from build123d import *

# Parameters (mm, degrees)
F0_W     = 103.5
F0_H     = 78.5
F0_R     = 10
F1_DEPTH = 18
F2_DEPTH = 7


with BuildPart() as f1:
    # F0 (on Top) → F1 (new body)
    with BuildSketch(Plane.XY):
        Rectangle(F0_W, F0_H)
        with Locations((-36, -24)):
            Circle(F0_R, mode=Mode.SUBTRACT)
        with Locations((-12, -24)):
            Circle(F0_R, mode=Mode.SUBTRACT)
        with Locations((12, -24)):
            Circle(F0_R, mode=Mode.SUBTRACT)
        with Locations((36, -24)):
            Circle(F0_R, mode=Mode.SUBTRACT)
        with Locations((-36, 0)):
            Circle(F0_R, mode=Mode.SUBTRACT)
        with Locations((-12, 0)):
            Circle(F0_R, mode=Mode.SUBTRACT)
        with Locations((-36, 24)):
            Circle(F0_R, mode=Mode.SUBTRACT)
        with Locations((-12, 24)):
            Circle(F0_R, mode=Mode.SUBTRACT)
        with Locations((12, 0)):
            Circle(F0_R, mode=Mode.SUBTRACT)
        with Locations((36, 0)):
            Circle(F0_R, mode=Mode.SUBTRACT)
        with Locations((12, 24)):
            Circle(F0_R, mode=Mode.SUBTRACT)
        with Locations((36, 24)):
            Circle(F0_R, mode=Mode.SUBTRACT)
    extrude(amount=F1_DEPTH)

    # F0 (on Top) → F2 (join)
    with BuildSketch(Plane.XY):
        Rectangle(F0_W, F0_H)
        with Locations((-36, -24)):
            Circle(F0_R, mode=Mode.SUBTRACT)
        with Locations((-12, -24)):
            Circle(F0_R, mode=Mode.SUBTRACT)
        with Locations((12, -24)):
            Circle(F0_R, mode=Mode.SUBTRACT)
        with Locations((36, -24)):
            Circle(F0_R, mode=Mode.SUBTRACT)
        with Locations((-36, 0)):
            Circle(F0_R, mode=Mode.SUBTRACT)
        with Locations((-12, 0)):
            Circle(F0_R, mode=Mode.SUBTRACT)
        with Locations((-36, 24)):
            Circle(F0_R, mode=Mode.SUBTRACT)
        with Locations((-12, 24)):
            Circle(F0_R, mode=Mode.SUBTRACT)
        with Locations((12, 0)):
            Circle(F0_R, mode=Mode.SUBTRACT)
        with Locations((36, 0)):
            Circle(F0_R, mode=Mode.SUBTRACT)
        with Locations((12, 24)):
            Circle(F0_R, mode=Mode.SUBTRACT)
        with Locations((36, 24)):
            Circle(F0_R, mode=Mode.SUBTRACT)
        with Locations((-36, -24)):
            Circle(F0_R)
        with Locations((-12, -24)):
            Circle(F0_R)
        with Locations((12, -24)):
            Circle(F0_R)
        with Locations((36, -24)):
            Circle(F0_R)
        with Locations((12, 0)):
            Circle(F0_R)
        with Locations((-12, 0)):
            Circle(F0_R)
        with Locations((-36, 0)):
            Circle(F0_R)
        with Locations((-36, 24)):
            Circle(F0_R)
        with Locations((-12, 24)):
            Circle(F0_R)
        with Locations((12, 24)):
            Circle(F0_R)
        with Locations((36, 24)):
            Circle(F0_R)
        with Locations((36, 0)):
            Circle(F0_R)
    extrude(amount=-F2_DEPTH)


solid = f1.part
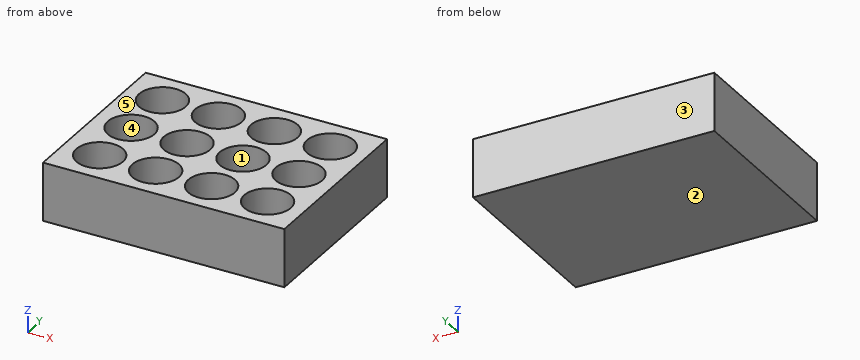
For this review, take the finished solid that the model builds, in its own axes (mm). Face numbers are marked on the shaded views. A direction names the side the tool comes from. Round coordinates to 2 decimals unless told otherwise and drop trailing zeros. Loops run counter-clockwise (first coordinate to the right, second up) from the corner with the lowest first, then second, coordinate; pieces in that order, holes last. Notation, with made-up numbers: (67, 31.5) - (124, 31.5) arc R28 ccw to (124, 68.5) - close; hole circle Ø9 at (-7, -16.75). An arc over 180 degrees is marked (long way). One line per item, written item: value. Start each with the question number.
Item 1: For L1, parallel to Y at x = -12, z = 5.75; L2, parallel to Y at x = -41.5, z = 2.5; L3, parallel to X at y = -5, z = 8, list the stretches that pass through material, from the lowest coordinate up.
Item 2: Take a section at A-A (z = 13). State how many separate pieces and enclosed holes the cut face has, plus the area to 3 significant figures.
Item 3: For the marked faces 1 and 2, list the 3-axis set-ups (+Z, -Z, +X, -X, +Y, -Y) from which the entire face can be reached by the end or side of a thin tool; tool diameter is ignored.
Item 4: Take a section at D-D (y = -32). Give the boundary of the cut face in (x, z), plus the area to 3 significant figures.
Item 5: Take a section at B-B (x = -12). Give the boundary of the cut face in (y, z).
Item 6: The part is to be moulded in two halves that separate along Y. For the marked faces 3, 4 and 5, say which applies: +Y half, -Y half, draft (parallel to the pull), parting line (faces both ways), or undercut.
Item 7: Take a section at C-C (y = -24). Give the boundary of the cut face in (x, z), plus the area to 3 significant figures.
Item 8: Clearance check with a flat-ended pin moving along its axis: pin 1 Ø16 at (x, y) = (-12, -24) entering from +Z. State where the tip first meets the part, or that it passes through.
Answer below:
1. L1: y = -39.25 to -34, -14 to -10, 10 to 14, 34 to 39.25
1. L2: y = -39.25 to -32.35, -15.65 to -8.35, 8.35 to 15.65, 32.35 to 39.25
1. L3: x = -51.75 to -44.66, -27.34 to -20.66, -3.34 to 3.34, 20.66 to 27.34, 44.66 to 51.75
2. separate pieces: 1
2. enclosed holes: 12
2. area: 4,350 mm2
3. face 1: +Z
3. face 2: -Z, +X, -X, +Y, -Y
4. outline: (-51.75, -7) - (51.75, -7) - (51.75, 18) - (42, 18) - (42, 0) - (30, 0) - (30, 18) - (18, 18) - (18, 0) - (6, 0) - (6, 18) - (-6, 18) - (-6, 0) - (-18, 0) - (-18, 18) - (-30, 18) - (-30, 0) - (-42, 0) - (-42, 18) - (-51.75, 18) - close
4. area: 1,720 mm2
5. outline: (-39.25, -7) - (39.25, -7) - (39.25, 18) - (34, 18) - (34, 0) - (14, 0) - (14, 18) - (10, 18) - (10, 0) - (-10, 0) - (-10, 18) - (-14, 18) - (-14, 0) - (-34, 0) - (-34, 18) - (-39.25, 18) - close
6. face 3: +Y half
6. face 4: undercut
6. face 5: draft
7. outline: (-51.75, -7) - (51.75, -7) - (51.75, 18) - (46, 18) - (46, 0) - (26, 0) - (26, 18) - (22, 18) - (22, 0) - (2, 0) - (2, 18) - (-2, 18) - (-2, 0) - (-22, 0) - (-22, 18) - (-26, 18) - (-26, 0) - (-46, 0) - (-46, 18) - (-51.75, 18) - close
7. area: 1,150 mm2
8. pin 1: stops at z = 0
